Autodesk Inventor part; units mm, degrees
ref_plane "YZ Plane" through (0, 0, 0) normal (1, 0, 0) x (0, 1, 0)
ref_plane "XZ Plane" through (0, 0, 0) normal (0, 1, 0) x (-1, 0, 0)
ref_plane "XY Plane" through (0, 0, 0) normal (0, 0, 1) x (1, 0, 0)
sketch "Skizze1" plane through (0, 0, 0) normal (0, 0, 1) x (1, 0, 0)
  line L0 (-52.5, 39) -> (52.5, 39)
  line L1 (-52.5, -39) -> (52.5, -39)
  line L2 (52.5, -39) -> (52.5, -43.25)
  line L3 (-52.5, -39) -> (-52.5, -43.25)
  line L4 (-60.5, -43.25) -> (-60.5, 43.25)
  line L5 (-52.5, 39) -> (-52.5, 43.25)
  line L6 (52.5, 39) -> (52.5, 43.25)
  line L7 (60.5, 43.25) -> (60.5, -43.25)
  arc A0 (-52.5, 43.25) -> (-60.5, 43.25) centre (-56.5, 43.25) ccw
  arc A1 (60.5, 43.25) -> (52.5, 43.25) centre (56.5, 43.25) ccw
  arc A2 (52.5, -43.25) -> (60.5, -43.25) centre (56.5, -43.25) ccw
  arc A3 (-60.5, -43.25) -> (-52.5, -43.25) centre (-56.5, -43.25) ccw
  line L8 (0, 66.15) -> (0, -66.15) construction
  line L9 (-84.7, 0) -> (84.7, 0) construction
  circle A4 centre (-56.5, 43.25) radius 1.4
  circle A5 centre (56.5, 43.25) radius 1.4
  circle A6 centre (56.5, -43.25) radius 1.4
  circle A7 centre (-56.5, -43.25) radius 1.4
  point P0 (0, 0)
  dimension "d0" = 121
  dimension "d1" = 78
  dimension "d2" = 8
  dimension "d3" = 86.5
  dimension "d4" = 2.8
extrude "Extrusion1" add sketch "Skizze1" along normal blind 1.1
sketch "Skizze8" plane through (0, 0, 1.1) normal (0, 0, 1) x (1, 0, 0)
  line L0 (-58.5, -37) -> (58.5, -37)
  line L1 (58.5, -37) -> (58.5, 37)
  line L2 (58.5, 37) -> (-58.5, 37)
  line L3 (-58.5, 37) -> (-58.5, -37)
  line L4 (-58.5, -37) -> (58.5, 37) construction
  line L5 (58.5, -37) -> (-58.5, 37) construction
  line L6 (60.5, -43.25) -> (60.5, 43.25)
  line L7 (52.5, 39) -> (-52.5, 39)
  line L8 (-60.5, 43.25) -> (-60.5, -43.25)
  arc A0 (-60.5, -43.25) -> (-52.5, -43.25) centre (-56.5, -43.25) ccw
  line L9 (-52.5, -43.25) -> (-52.5, -39)
  line L10 (-52.5, -39) -> (52.5, -39)
  line L11 (52.5, -39) -> (52.5, -43.25)
  arc A1 (52.5, -43.25) -> (60.5, -43.25) centre (56.5, -43.25) ccw
  line L12 (60.5, -43.25) -> (60.5, 43.25)
  arc A2 (60.5, 43.25) -> (52.5, 43.25) centre (56.5, 43.25) ccw
  line L13 (52.5, 43.25) -> (52.5, 39)
  line L14 (52.5, 39) -> (-52.5, 39)
  line L15 (-52.5, 39) -> (-52.5, 43.25)
  arc A3 (-52.5, 43.25) -> (-60.5, 43.25) centre (-56.5, 43.25) ccw
  circle A4 centre (-56.5, -43.25) radius 1.4
  circle A5 centre (56.5, -43.25) radius 1.4
  circle A6 centre (56.5, 43.25) radius 1.4
  circle A7 centre (-56.5, 43.25) radius 1.4
  point P0 (0, 0)
  dimension "d45" = 2
  dimension "d46" = 2
extrude "Extrusion8" add sketch "Skizze8" along normal blind 5.4
sketch "Skizze9" plane through (-52.5, 39, 0) normal (0, 1, 0) x (1, 0, 0)
  line L0 (105, -6.5) -> (0, -6.5)
  line L1 (-6, -6.5) -> (111, -6.5)
  line L2 (99.9, -6.5) -> (94.5, -6.5)
  line L3 (94.5, -6.5) -> (94.5, -4.1)
  line L4 (94.5, -4.1) -> (99.9, -4.1)
  line L5 (99.9, -4.1) -> (99.9, -6.5)
  line L6 (86.95, -6.5) -> (78.95, -6.5)
  line L7 (78.95, -6.5) -> (78.95, -3.5)
  line L8 (78.95, -3.5) -> (86.95, -3.5)
  line L9 (86.95, -3.5) -> (86.95, -6.5)
  line L10 (68.25, -6.5) -> (60.25, -6.5)
  line L11 (60.25, -6.5) -> (60.25, -3.5)
  line L12 (60.25, -3.5) -> (68.25, -3.5)
  line L13 (68.25, -3.5) -> (68.25, -6.5)
  line L14 (53.5, -6.5) -> (37.9, -6.5)
  line L15 (37.9, -6.5) -> (37.9, 0.5)
  line L16 (37.9, 0.5) -> (53.5, 0.5)
  line L17 (53.5, 0.5) -> (53.5, -6.5)
  line L18 (20.2, -6.5) -> (27.2, -6.5)
  line L19 (27.2, -6.5) -> (27.2, -1.1)
  line L20 (27.2, -1.1) -> (20.2, -1.1)
  line L21 (20.2, -1.1) -> (20.2, -6.5)
  line L22 (97.2, -4.1) -> (97.2, -6.5) construction
  line L23 (82.95, -3.5) -> (82.95, -6.5) construction
  line L24 (64.25, -3.5) -> (64.25, -6.5) construction
  line L25 (45.7, 0.5) -> (45.7, -6.5) construction
  line L26 (23.7, -1.1) -> (23.7, -6.5) construction
  line L27 (105, 0) -> (105, -6.5) construction
  line L28 (37.9, -6.5) -> (27.2, -6.5)
  line L29 (27.2, -6.5) -> (27.2, -5.5)
  line L30 (27.2, -5.5) -> (37.9, -5.5)
  line L31 (37.9, -5.5) -> (37.9, -6.5)
  point P0 (52.5, 0)
  point P1 (27.2, -6.5)
  point P2 (94.5, -6.5)
  point P3 (99.9, -6.5)
  dimension "d49" = 7.8
  dimension "d50" = 22.05
  dimension "d51" = 40.75
  dimension "d52" = 59.3
  dimension "d53" = 81.3
  dimension "d54" = 2.4
  dimension "d55" = 3
  dimension "d56" = 7
  dimension "d57" = 5.4
  dimension "d58" = 5.4
  dimension "d59" = 8
  dimension "d60" = 8
  dimension "d61" = 15.6
  dimension "d62" = 7
  dimension "d65" = 1
extrude "Extrusion9" cut sketch "Skizze9" against normal blind 12
sketch "Skizze11" plane through (0, 0, 1.1) normal (0, 0, 1) x (1, 0, 0)
  line L0 (-58.5, 37) -> (-32.3, 37)
  line L1 (-37.5, 37) -> (-47.5, 37)
  line L2 (-47.5, 37) -> (-47.5, 17)
  line L3 (-47.5, 17) -> (-37.5, 17)
  line L4 (-37.5, 17) -> (-37.5, 37)
  line L5 (-52.5, 39) -> (-52.5, 43.25)
  point P0 (0, 0)
  point P1 (-42.5, 37)
  dimension "d66" = 10
  dimension "d67" = 10
  dimension "d68" = 20
extrude "Extrusion10" add sketch "Skizze11" along normal blind 3.6
sketch "Skizze12" plane through (-52.5, 39, 6.5) normal (0, 1, 0) x (1, 0, 0)
  line L0 (5, 5.4) -> (5, 1.8)
  line L1 (15, 5.4) -> (5, 5.4)
  line L2 (15, 5.4) -> (15, 1.8)
  line L3 (10, 5.4) -> (10, 0) construction
  line L4 (13.6, 5) -> (11.4, 5)
  line L5 (11.4, 5) -> (11.4, 2.8)
  line L6 (11.4, 2.8) -> (13.6, 2.8)
  line L7 (13.6, 2.8) -> (13.6, 5)
  line L8 (13.6, 5) -> (11.4, 2.8) construction
  line L9 (11.4, 5) -> (13.6, 2.8) construction
  line L10 (8.6, 5) -> (6.4, 5)
  line L11 (6.4, 5) -> (6.4, 2.8)
  line L12 (6.4, 2.8) -> (8.6, 2.8)
  line L13 (8.6, 2.8) -> (8.6, 5)
  line L14 (8.6, 5) -> (6.4, 2.8) construction
  line L15 (6.4, 5) -> (8.6, 2.8) construction
  line L16 (5, 1.8) -> (15, 1.8)
  point P0 (52.5, 6.5)
  point P1 (12.5, 3.9)
  point P2 (7.5, 3.9)
  point P3 (7.5, 3.9)
  point P4 (12.5, 3.9)
  point P5 (8.6, 5.4)
  point P6 (6.4, 5.4)
  point P7 (13.6, 5.4)
  point P8 (11.4, 5.4)
  point P9 (7.5, 3.9)
  dimension "d73" = 5
  dimension "d74" = 2.2
  dimension "d75" = 2.2
  dimension "d78" = 1.5
extrude "Extrusion11" cut sketch "Skizze12" against normal up to surface (22 mm away) contours L7 L6 L5 L4 | L13 L12 L11 L10
sketch "Skizze13" plane through (-52.5, 39, 6.5) normal (0, 1, 0) x (1, 0, 0)
  line L0 (13.6, 2.8) -> (11.4, 2.8) construction
  line L1 (11.4, 5) -> (13.6, 5) construction
  line L2 (8.6, 2.8) -> (6.4, 2.8) construction
  line L3 (6.4, 5) -> (8.6, 5) construction
  line L4 (7.5, 2.8) -> (7.5, 5) construction
  line L5 (8.6, 5) -> (6.4, 5) construction
  line L6 (12.5, 5) -> (12.5, 2.8) construction
  line L7 (14, 5.4) -> (11, 5.4)
  line L8 (11, 5.4) -> (11, 2.4)
  line L9 (11, 2.4) -> (14, 2.4)
  line L10 (14, 2.4) -> (14, 5.4)
  line L11 (14, 5.4) -> (11, 2.4) construction
  line L12 (11, 5.4) -> (14, 2.4) construction
  line L13 (9, 5.4) -> (6, 5.4)
  line L14 (6, 5.4) -> (6, 2.4)
  line L15 (6, 2.4) -> (9, 2.4)
  line L16 (9, 2.4) -> (9, 5.4)
  line L17 (9, 5.4) -> (6, 2.4) construction
  line L18 (6, 5.4) -> (9, 2.4) construction
  point P0 (52.5, 6.5)
  point P1 (12.5, 3.9)
  point P2 (7.5, 3.9)
  dimension "d79" = 3
  dimension "d80" = 3
  dimension "d81" = 3
  dimension "d82" = 3
extrude "Extrusion12" cut sketch "Skizze13" against normal blind 10
equation "\"d60\" = d59"
properties part number "Display 5inch Housing"
Could you check a few things on this model? Use its own coordinates, in mm. A direction names the side the tool comes from. Give positions to 0.01 mm unless a question says otherwise; leave off trailing zeros. Write each loop counter-clockwise with the first axis right and the second up, starting at its lowest first coordinate (ties: lowest second). Pieces come first, ordered by that corner, then holes. Notation, with made-up numbers: (75, 6) - (96, 6) arc R17 cw to (96, 16) - close; hole circle Ø1 at (38, -4.75). An arc over 180 degrees is marked (long way). One line per item, written item: value. Start each with the question number.
Item 1: Please list where these lines run through material, in increasing order: line 1 (Y direction, x = -56.5, z = 2.75); line 2 (Y direction, x = -51, z = 1.75); line 3 (X direction, y = -28, z = 5). Write a range as from..to.
Item 2: Imagine slicing it at A-A, the plane x = -56.5. List the corners of the cut face in (y, z) for me, and give its area (3 significant figures).
Item 3: Imagine slicing it at D-D, the plane z = 2.5. Give the number of separate pieces and of enclosed holes in the cut face, and give its area (3 significant figures).
Item 4: Which directions (+Z, -Z, +X, -X, +Y, -Y) give clear straight access to the entire face, cutting with the end or side of a thin tool? Please do faces 1 (the face through (-45, 29, 3.9)), 2 (the face through (58.5, -1, 4)), 3 (the face through (-14.6, 35.8, 0.3)).
Item 5: I'm going to push flat-ended pins straight in: pin 1 (0.9 mm diameter, centred on x = -45, z = 2.5, fed in from +Y); pin 2 (0.6 mm diameter, centred on x = 30, y = 38, fed in from +Z); pin 3 (3 mm diameter, centred on x = -44.5, y = 19.5, fed in from +Z). Where does each tip first touch, or does it pass through?
Item 6: Imagine slicing it at C-C, the plane y = 19. List the corners of the cut face in (x, z) for me.
Item 7: Imagine slicing it at B-B, the plane y = -17. List the corners of the cut face in (x, z) for me, and give its area (3 significant figures).
Geometry says:
1. line 1: -47.25..-44.65, -41.85..-37, 37..41.85, 44.65..47.25
1. line 2: -39..-37, 37..39
1. line 3: -60.5..-58.5, 58.5..60.5
2. outline: (-47.25, 0) - (-44.65, 0) - (-44.65, 6.5) - (-47.25, 6.5) - close; (-41.85, 0) - (41.85, 0) - (41.85, 6.5) - (37, 6.5) - (37, 1.1) - (-37, 1.1) - (-37, 6.5) - (-41.85, 6.5) - close; (44.65, 0) - (47.25, 0) - (47.25, 6.5) - (44.65, 6.5) - close
2. area: 178 mm^2
3. separate pieces: 4
3. enclosed holes: 4
3. area: 1,030 mm^2
4. face 1: +Y
4. face 2: +Z
4. face 3: +Z, -Z, +Y
5. pin 1: y = -37
5. pin 2: z = 3.5
5. pin 3: z = 4.7
6. outline: (-60.5, 0) - (60.5, 0) - (60.5, 6.5) - (58.5, 6.5) - (58.5, 1.1) - (-37.5, 1.1) - (-37.5, 4.7) - (-47.5, 4.7) - (-47.5, 1.1) - (-58.5, 1.1) - (-58.5, 6.5) - (-60.5, 6.5) - close; hole (-46.1, 1.5) - (-43.9, 1.5) - (-43.9, 3.7) - (-46.1, 3.7) - close; hole (-41.1, 1.5) - (-38.9, 1.5) - (-38.9, 3.7) - (-41.1, 3.7) - close
7. outline: (-60.5, 0) - (60.5, 0) - (60.5, 6.5) - (58.5, 6.5) - (58.5, 1.1) - (-58.5, 1.1) - (-58.5, 6.5) - (-60.5, 6.5) - close
7. area: 155 mm^2
